Can you work these out from the model? Positions are in its coordinate system, mm. Face numbers are marked on the shaded views. Round coordinates to 2 decimals unless told otherwise and drop trailing zeros. Loops run counter-clockwise (first coordinate to the right, second up) from the corner with the lowest first, then second, coordinate; pieces in that order, holes last. Notation, with made-up numbers: (49, 19.25) -> (66, 19.25) arc R18 cw to (66, 40.25) -> close; hole circle Ø4 at (8.5, 57.5). An arc over 180 degrees is marked (long way). Answer as a JSON object with one key per item and string values.
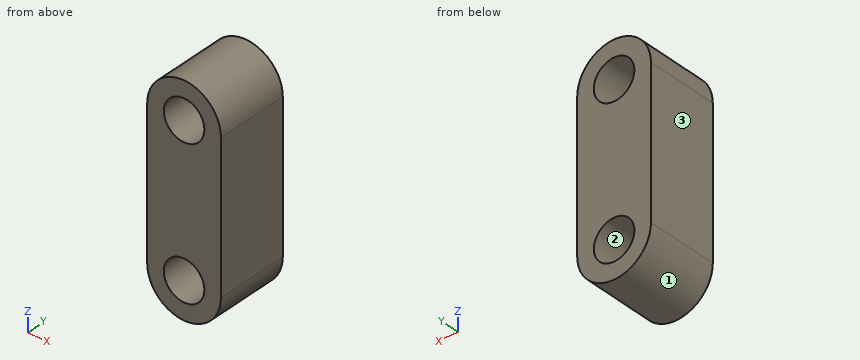
```python
from build123d import *

# Parameters (mm, degrees)
SKETCH3_R           = 2.75
BOSS_EXTRUDE1_DEPTH = 10


with BuildPart() as part:
    # Sketch3 → Boss-Extrude1 (new body)
    with BuildSketch(Plane(origin=(0, 0, 0), x_dir=(1, 0, 0), z_dir=(0, 1, 0))):
        with BuildLine():
            ThreePointArc((-5, 0), (0, -5), (5, 0))
            Line((5, 0), (5, 20))
            ThreePointArc((5, 20), (0, 25), (-5, 20))
            Line((-5, 20), (-5, 0))
        make_face()
        Circle(SKETCH3_R, mode=Mode.SUBTRACT)
        with Locations((0, 20)):
            Circle(SKETCH3_R, mode=Mode.SUBTRACT)
    extrude(amount=BOSS_EXTRUDE1_DEPTH)


solid = part.part
```
Q1. If I drill on L1, parallel to Z at x = 0, y = 3.5; L2, parallel to Z at x = 2, y = 4.5; L3, parallel to X at y = 5.75, z = -20, over which ranges is the centre line in solid material (lowest first)? Write a range as [from, to].
Determined:
{"L1": "[-25, -22.75], [-17.25, -2.75], [2.75, 5]", "L2": "[-24.58, -21.89], [-18.11, -1.89], [1.89, 4.58]", "L3": "[-5, -2.75], [2.75, 5]"}
Q2. I want a section at B-B, the plane z = -22.25. Write out the boundary of the cut face in (x, y), then the cut area to 3 significant figures.
Determined:
{"outline": "(-4.47, 0) -> (-1.58, 0) -> (-1.58, 10) -> (-4.47, 10) -> close; (1.58, 0) -> (4.47, 0) -> (4.47, 10) -> (1.58, 10) -> close", "area": "57.7 mm²"}
Q3. We'd pull the mould along Z, two halves only. Please class the marked faces 1, 2 and 3: pulls with the +Z half, pulls with the -Z half, needs draft (parallel to the pull), parting line crosses it, or undercut.
Determined:
{"face 1": "pulls with the -Z half", "face 2": "undercut", "face 3": "needs draft"}
Q4. I want a section at A-A, the plane x = 0. Write out the boundary of the cut face in (y, z), then the cut area to 3 significant figures.
Determined:
{"outline": "(0, -25) -> (10, -25) -> (10, -22.75) -> (0, -22.75) -> close; (0, -17.25) -> (10, -17.25) -> (10, -2.75) -> (0, -2.75) -> close; (0, 2.75) -> (10, 2.75) -> (10, 5) -> (0, 5) -> close", "area": "190 mm²"}
Q5. I want a section at C-C, the plane y = 1.75. Write out the boundary of the cut face in (x, z), then the cut area to 3 significant figures.
Determined:
{"outline": "(-5, -20) arc R5 ccw to (5, -20) -> (5, 0) arc R5 ccw to (-5, 0) -> close; hole circle Ø5.5 at (0, -20); hole circle Ø5.5 at (0, 0)", "area": "231 mm²"}
Q6. I want a section at D-D, the plane x = 1.25. Write out the boundary of the cut face in (y, z).
Determined:
{"outline": "(0, -24.84) -> (10, -24.84) -> (10, -22.45) -> (0, -22.45) -> close; (0, -17.55) -> (10, -17.55) -> (10, -2.45) -> (0, -2.45) -> close; (0, 2.45) -> (10, 2.45) -> (10, 4.84) -> (0, 4.84) -> close"}
Q7. I'm going to push flat-ended pins straight in: pin 1 (5 mm diameter, centred on x = -4, y = 3, fed in from +Z); pin 2 (3 mm diameter, centred on x = 3, y = 3.5, fed in from -Z); pin 3 (4.5 mm diameter, centred on x = 0, z = 0, fed in from -Y). Where does each tip first touch, or does it pass through?
Determined:
{"pin 1": "z = 4.77", "pin 2": "z = -24.77", "pin 3": "through"}
